For this review, take the finished solid that the model builds, in its own axes (mm). A direction names the side the tool comes from. Give positions to 0.01 mm unless a question says otherwise; leave off trailing zeros. Order: outer loops, then holes, each group sorted by start corner. A loop starts at its lowest first (then second) coordinate and runs counter-clockwise, first axis right, second up. Notation, with made-up numbers: (78, 63.5) -> (100, 63.5) arc R13 ccw to (100, 88.5) -> close; hole circle Ø1 at (87, 12.25). An arc over 180 degrees is marked (long way). Return JSON: item names as keys, results as strings. Group by question number.
1) Add section B-B (z = 0). Give the boundary of the cut face in (x, y), then the cut area to 3 significant figures.
2) Add section C-C (y = 1). Give the boundary of the cut face in (x, z).
3) The part is to be moulded in two halves that separate along Y. For faces 1 (the face through (-1.1, -5, 2.3)), 2 (the face through (5, -4, 1.6)), 3 (the face through (2.23, -5.99, -0.29)), 4 (the face through (-1.8, -3, -5.1)), say which applies: released by +Y, released by -Y, zero draft, split by the parting line, or undercut.
4) Insertion check: P1, Ø1, axis at x = 4.5, z = -1, coming from the -Y side; P2, Ø6, axis at y = -11, z = 3, coming from the +X side; P3, Ø1.5, axis at y = 1, z = 0, coming from the -X side; P4, Ø1, axis at x = -0.5, y = -13, coming from the +Z side. Each pin has a flat end and moves straight along its axis. Give the tip position at first contact, or say it passes through.
5) To check wall thickness, follow line 1 along Y through (x, z) = (2.75, 0); line 2 along Z through (x, y) = (-0.25, 1); line 3 along Y through (x, z) = (2.5, 2). State the ranges of each line that lie inside material, in increasing order.
6) Add section D-D (x = 4.5). State how many separate pieces and enclosed holes the cut face has, then the cut area to 3 significant figures.
7) Add section A-A (x = 0). Give the boundary of the cut face in (y, z).
8) For faces 5 (the face through (-2, -7, 2)), 6 (the face through (0, 3, 0)), 7 (the face through (-3.78, -12.32, -2.9)), list the 3-axis set-ups (+Z, -Z, +X, -X, +Y, -Y) from which the entire face can be reached by the end or side of a thin tool; tool diameter is ignored.
Autodesk Inventor part; units mm, degrees
ref_plane "YZ Plane" through (0, 0, 0) normal (1, 0, 0) x (0, 1, 0)
ref_plane "XZ Plane" through (0, 0, 0) normal (0, 1, 0) x (-1, 0, 0)
ref_plane "XY Plane" through (0, 0, 0) normal (0, 0, 1) x (1, 0, 0)
sketch "Sketch3" plane through (0, 0, 0) normal (0, 0, 1) x (1, 0, 0)
  line L0 (0, 3) -> (7.5, 3)
  line L1 (7.5, 3) -> (7.5, -3)
  line L2 (7.5, -3) -> (5.25, -3)
  line L3 (5.25, -3) -> (5.25, -5)
  line L4 (5.25, -5) -> (4.7625, -5)
  line L5 (0, -21.6) -> (0, 7.1)
  line L6 (4.7625, -5) -> (4.7625, -17.5)
  line L7 (4.7625, -17.5) -> (0, -17.5)
  point P0 (0, 0)
  point P1 (7.5, 0)
  dimension "d6" = 6
  dimension "d7" = 15
  dimension "d8" = 10.5
  dimension "d9" = 2
  dimension "d11" = 9.525
  dimension "d12" = 12.5
revolve "Revolution1" add sketch "Sketch3" angle 360 about axis through (0, -10, 0) along (0, 1, 0)
sketch "Sketch4" plane through (0, 0, 0) normal (1, 0, 0) x (0, 1, 0)
  circle A0 centre (1, 0) radius 1.25
  line L0 (3, 7.5) -> (3, -7.5)
  point P0 (0, 0)
  dimension "d13" = 2.5
  dimension "d14" = 2
extrude "Extrusion3" cut sketch "Sketch4" along normal through all both and the other way through all
sketch "Sketch5" plane through (0, 0, 0) normal (1, 0, 0) x (0, 1, 0)
  line L0 (-7, 2.25) -> (-5, 2.25)
  line L1 (-5, 2.25) -> (-5, 4.7625)
  line L2 (-5, 4.7625) -> (-7, 4.7625)
  line L3 (-7, 4.7625) -> (-7, 2.25)
  line L4 (-5, 4.7625) -> (-17.5, 4.7625)
  line L5 (-5, 5.25) -> (-5, -5.25)
  line L6 (-21, 0) -> (3.5, 0)
  point P0 (0, 0)
  dimension "d17" = 2
  dimension "d18" = 4.5
revolve "Revolution2" cut sketch "Sketch5" angle 360 about axis through (0, -10, 0) along (0, 1, 0)
thread "Thread1"
chamfer "Chamfer1" distance 0.5 angle 45 2 edges at (-4.7625, -17.5, 0) (-4.7625, -7, 0)
properties part number "Thumb Screw" material "Steel, Mild"
Evaluation:
{
 "1": {"outline": "(-7.5, -3) -> (-5.25, -3) -> (-5.25, -5) -> (-2.25, -5) -> (-2.25, -7) -> (-4.26, -7) -> (-4.76, -7.5) -> (-4.76, -17) -> (-4.26, -17.5) -> (4.26, -17.5) -> (4.76, -17) -> (4.76, -7.5) -> (4.26, -7) -> (2.25, -7) -> (2.25, -5) -> (5.25, -5) -> (5.25, -3) -> (7.5, -3) -> (7.5, -0.25) -> (-7.5, -0.25) -> close; (-7.5, 2.25) -> (7.5, 2.25) -> (7.5, 3) -> (-7.5, 3) -> close", "area": "182 mm^2"},
 "2": {"outline": "(-7.4, -1.25) arc R7.5 ccw to (7.4, -1.25) -> close; (-7.4, 1.25) -> (7.4, 1.25) arc R7.5 ccw to start"},
 "3": {"face 1": "undercut", "face 2": "zero draft", "face 3": "undercut", "face 4": "released by -Y"},
 "4": {"P1": "y = -17.5", "P2": "x = 4.76", "P3": "through", "P4": "z = 4.76"},
 "5": {"line 1": "-17.5 to -7, -5 to -0.25, 2.25 to 3", "line 2": "-7.5 to -1.25, 1.25 to 7.5", "line 3": "-17.5 to -7, -5 to 3"},
 "6": {"separate pieces": "2", "enclosed holes": "1", "area": "109 mm^2"},
 "7": {"outline": "(-17.5, -4.26) -> (-17, -4.76) -> (-7.5, -4.76) -> (-7, -4.26) -> (-7, -2.25) -> (-5, -2.25) -> (-5, -5.25) -> (-3, -5.25) -> (-3, -7.5) -> (3, -7.5) -> (3, 7.5) -> (-3, 7.5) -> (-3, 5.25) -> (-5, 5.25) -> (-5, 2.25) -> (-7, 2.25) -> (-7, 4.26) -> (-7.5, 4.76) -> (-17, 4.76) -> (-17.5, 4.26) -> close; hole circle Ø2.5 at (1, 0)"},
 "8": {"face 5": "none", "face 6": "+Z, -Z, +X, -X, +Y", "face 7": "-Y"}
}
